```python
from build123d import *

# Parameters (mm, degrees)
F1_DEPTH = 41.275
F2_R     = 1.6
F2_R_2   = 1.25
F3_DEPTH = 4.6024929371
F4_DEPTH = 9.3840608367
F6_R     = 10.16
F7_R     = 2.54


with BuildPart() as f1:
    # F0 (on Front) → F1 (new body)
    with BuildSketch(Plane.XZ):
        Polygon((-10.9985226281, 6.35), (0, 0), (3.1994554543, 0), (3.0682228412, 1.200819531), (11.1481153525, 2.0838376541), (11.2019242694, 1.5914692042), (20.7514773719, 2.6351004709), (20.7514773719, 6.35), (1.7014773719, 6.35), (-84.8131810245, 56.299261314), (-87.9881810245, 50.8), align=None)
        with BuildLine():
            Line((3.1994554543, 0), (0, 0))
            Line((0, 0), (-10.9985226281, 6.35))
            ThreePointArc((-10.9985226281, 6.35), (3.7335153721, -2.5398099993), (20.7514773719, 0))
            Line((20.7514773719, 0), (10.7844894565, 0))
            Line((10.7844894565, 0), (3.2889773719, -0.8191535968))
            Line((3.2889773719, -0.8191535968), (3.1994554543, 0))
        make_face()
        Polygon((10.7844894565, 0), (20.7514773719, 0), (20.7514773719, 1.5875), (11.3150609664, 0.5562329762), (11.3688698832, 0.0638645263), align=None)
    extrude(amount=F1_DEPTH)

    # F2 (on face) → F3 (cut, through all)
    with BuildSketch(Plane.XY.offset(6.35)):
        with Locations((14.2388698832, -20.6375)):
            Circle(F2_R)
        with Locations((14.2388698832, -20.6375)):
            Circle(F2_R_2, mode=Mode.SUBTRACT)
        with Locations((14.2388698832, -20.6375)):
            Circle(F2_R_2)
    extrude(amount=-F3_DEPTH, mode=Mode.SUBTRACT)

    # F2 (on face) → F4 (cut, through all)
    with BuildSketch(Plane.XY.offset(6.35)):
        with Locations((14.2388698832, -20.6375)):
            Circle(F2_R_2)
    extrude(amount=-F4_DEPTH, mode=Mode.SUBTRACT)

    # F6
    f6_edges = [f1.edges().sort_by_distance(p)[0] for p in [
        (-10.998523, -20.6375, 6.35),
        (1.701477, -20.6375, 6.35),
    ]]
    fillet(f6_edges, radius=F6_R)

    # F7
    f7_edges = [f1.edges().sort_by_distance(p)[0] for p in [
        (-87.988181, -20.6375, 50.8),
        (-84.813181, -20.6375, 56.299261),
        (20.751477, -20.6375, 6.35),
    ]]
    fillet(f7_edges, radius=F7_R)


solid = f1.part
```
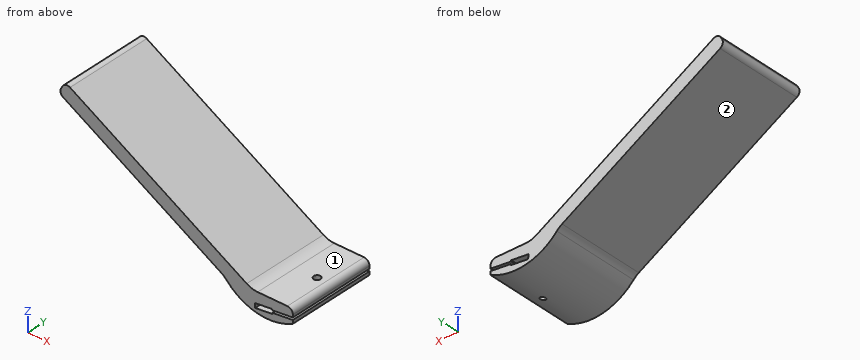
Could you check a few things on this model? Use its own coordinates, in mm. Face numbers are marked on the shaded views. A direction names the side the tool comes from. Coordinates: 2 decimals unless noted, no trailing zeros. Write each loop counter-clockwise with the first axis right and the second up, starting at its lowest first coordinate (ties: lowest second). Pieces come first, ordered by that corner, then holes. Notation, with made-up numbers: (56.5, 74.5) -> (70.5, 74.5) arc R21 ccw to (70.5, 101.5) -> close; hole circle Ø9 at (-28.5, 74.5). An arc over 180 degrees is marked (long way). Write item = value, one per line. Start each with the question number.
(1) Will these pins go through, and if not, where does the flat tip stop? pin 1 (10 mm diameter, centred on x = -42.5, y = -25.5, fed in from +Z); pin 2 (15 mm diameter, centred on x = 10, y = -14.5, fed in from +Z); pin 3 (3 mm diameter, centred on x = 14.24, y = -20.64, fed in from +Z).
(2) I need wall thicknesses on line 1 (Z direction, x = 9.5, y = -6); line 2 (Z direction, x = 14, y = -37); line 3 (Z direction, x = -47.5, y = -26). Which ranges of each line are inside material? Lowest first, please. Write a range as [from, to].
(3) I want a section at B-B (z = 20). Please give me the cut outline in (x, y) (3 decimals).
(4) I want a section at C-C (x = -64.5). Please give me the cut outline in (y, z) (3 decimals), plus the area to 3 significant figures.
(5) I want a section at A-A (y = -27.5). Please give me the cut outline in (x, z), plus the area to 3 significant figures.
(6) Which directions (+Z, -Z, +X, -X, +Y, -Y) give clear straight access to the entire face, cutting with the end or side of a thin tool? Please do the marked faces 1 and 2.
Result set:
q1.pin_1 = 34.76
q1.pin_2 = 6.53
q1.pin_3 = 1.04
q2.line_1 = [-3.02, -0.14], [1.9, 6.35]
q2.line_2 = [-2.48, 0.85], [1.9, 6.35]
q2.line_3 = [27.42, 34.76]
q3.outline = (-34.641, -41.275) -> (-21.941, -41.275) -> (-21.941, 0) -> (-34.641, 0) -> close
q4.outline = (-41.275, 37.239) -> (0, 37.239) -> (0, 44.571) -> (-41.275, 44.571) -> close
q4.area = 303 mm2
q5.outline = (-86.72, 53) arc R2.54 ccw to (-85.79, 49.53) -> (-12.48, 7.21) arc R10.16 cw to (-10.05, 5.25) arc R25.4 ccw to (20.75, 0) -> (20.75, 1.59) -> (11.32, 0.56) -> (11.37, 0.06) -> (3.29, -0.82) -> (3.07, 1.2) -> (11.15, 2.08) -> (11.2, 1.59) -> (20.75, 2.64) -> (20.75, 3.81) arc R2.54 ccw to (18.21, 6.35) -> (4.42, 6.35) arc R10.16 cw to (-0.66, 7.71) -> (-82.61, 55.03) arc R2.54 ccw to (-86.08, 54.1) -> close
q5.area = 799 mm2
q6.face_1 = +Z, +X, +Y, -Y
q6.face_2 = -Z, -X, +Y, -Y
